from build123d import *

# Parameters (mm, degrees)
SKETCH1_W           = 30
SKETCH1_H           = 7.6
BOSS_EXTRUDE1_DEPTH = 30
SKETCH2_R           = 11
CUT_EXTRUDE1_DEPTH  = 30
SKETCH3_W           = 50
SKETCH3_H           = 7.6
BOSS_EXTRUDE2_DEPTH = 3.5


with BuildPart() as part:
    # Sketch1 → Boss-Extrude1 (new body)
    with BuildSketch(Plane(origin=(0, 0, 0), x_dir=(1, 0, 0), z_dir=(0, 1, 0))):
        Rectangle(SKETCH1_W, SKETCH1_H)
    extrude(amount=BOSS_EXTRUDE1_DEPTH)

    # Sketch2 → Cut-Extrude1 (cut)
    with BuildSketch(Plane.XY.offset(3.8)):
        Polygon((-15, 30), (-15, 23), (-8, 30), align=None)
        Polygon((15, 30), (8, 30), (15, 23), align=None)
        with Locations((0, 15)):
            Circle(SKETCH2_R)
    extrude(amount=-CUT_EXTRUDE1_DEPTH, mode=Mode.SUBTRACT)

    # Sketch3 → Boss-Extrude2 (add)
    with BuildSketch(Plane.XZ):
        Rectangle(SKETCH3_W, SKETCH3_H)
    extrude(amount=-BOSS_EXTRUDE2_DEPTH)


solid = part.part
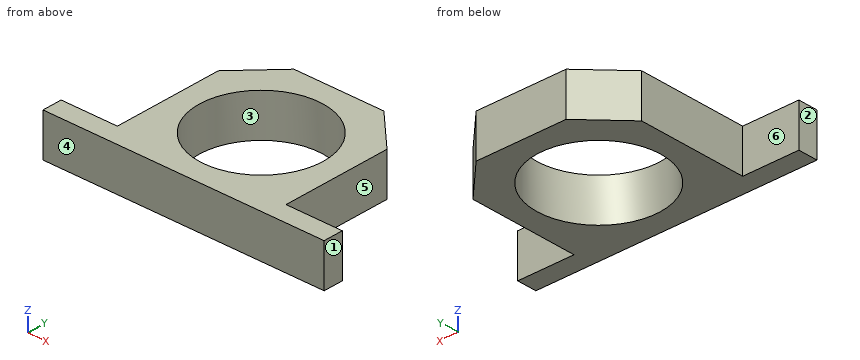
Geometry: final body of the model. Coordinates: model frame, mm. Face numbers are marked on the shaded views. A direction names the side the tool comes from. Give positions to 0.01 mm unless a question says otherwise; leave off trailing zeros. Write each loop counter-clockwise with the first axis right and the second up, starting at its lowest first coordinate (ties: lowest second). Pieces come first, ordered by that corner, then holes. Notation, with made-up numbers: (-9, -3) - (8, -3) arc R18 ccw to (8, 9) - close; hole circle Ø7 at (60, -17). An arc over 180 degrees is marked (long way). Return JSON: item names as keys, results as strings. Group by question number.
1) Section B-B on z = -2.25. Return the cut outline in (x, y), plus the area to 3 significant figures.
2) Set-up query: the marked faces 4, 5 and 6. Return all of +Z, -Z, +X, -X, +Y, -Y with unobstructed straight access to the full face (end or side cutting, diameter ignored); none if empty.
3) Section D-D on x = 12. Return the cut outline in (y, z), plus the area to 3 significant figures.
4) Line query: line 1 (Y direction, x = 0, z = 0.75); line 2 (X direction, y = 14.5, z = 0.5); line 3 (Y direction, x = 21.5, z = 3). Output: solid intervals per line, ascending.
5) Mould query, pull axis X, two halves, no side actions, for the marked faces 1, 2 and 3. Classes: released by +X, released by -X, zero draft, split by the parting line, or undercut.
6) Section A-A on y = 15. Return the cut outline in (x, z), plus the area to 3 significant figures.
7) Section C-C on x = 0. Return the cut outline in (y, z).
Filled in:
{
 "1": {"outline": "(-25, 0) - (25, 0) - (25, 3.5) - (15, 3.5) - (15, 23) - (8, 30) - (-8, 30) - (-15, 23) - (-15, 3.5) - (-25, 3.5) - close; hole circle Ø22 at (0, 15)", "area": "541 mm^2"},
 "2": {"face 4": "+Z, -Z, +X, -X, -Y", "face 5": "+Z, -Z, +X, +Y", "face 6": "+Z, -Z, -X, +Y"},
 "3": {"outline": "(0, -3.8) - (26, -3.8) - (26, 3.8) - (0, 3.8) - close", "area": "198 mm^2"},
 "4": {"line 1": "y = 0 to 4, 26 to 30", "line 2": "x = -15 to -10.99, 10.99 to 15", "line 3": "y = 0 to 3.5"},
 "5": {"face 1": "released by +X", "face 2": "released by -X", "face 3": "undercut"},
 "6": {"outline": "(-15, -3.8) - (-11, -3.8) - (-11, 3.8) - (-15, 3.8) - close; (11, -3.8) - (15, -3.8) - (15, 3.8) - (11, 3.8) - close", "area": "60.8 mm^2"},
 "7": {"outline": "(0, -3.8) - (4, -3.8) - (4, 3.8) - (0, 3.8) - close; (26, -3.8) - (30, -3.8) - (30, 3.8) - (26, 3.8) - close"}
}
